```python
from build123d import *

# Parameters (mm, degrees)
F0_R     = 10.1
F1_DEPTH = 10
F2_R     = 3.75
F3_DEPTH = 10


with BuildPart() as f1:
    # F0 (on Top) → F1 (new body)
    with BuildSketch(Plane.XY):
        Circle(F0_R)
    extrude(amount=F1_DEPTH)

    # F2 (on Top) → F3 (join)
    with BuildSketch(Plane.XY):
        Circle(F2_R)
    extrude(amount=-F3_DEPTH)

    # F4 (on Front) → F5 (revolve)
    with BuildSketch(Plane.XZ):
        with BuildLine():
            Line((-3.9404258132, 0), (-10.2904258132, 0))
            Line((-10.2904258132, 0), (-10.2904258132, -9.9157679855))
            Line((-10.2904258132, -9.9157679855), (-9.0434306607, -9.9157679855))
            ThreePointArc((-9.0434306607, -9.9157679855), (-8.3038120471, -4.0254245121), (-3.9404258132, 0))
        make_face()
    revolve(axis=Axis((0, 0, -4.4246494012), (0, 0, -1)))


solid = f1.part
```
For this review, take the finished solid that the model builds, in its own axes (mm). Give positions to 0.01 mm unless a question says otherwise; leave off trailing zeros. Write each loop counter-clockwise with the first axis right and the second up, starting at its lowest first coordinate (ties: lowest second). Pieces come first, ordered by that corner, then holes.
Item 1: Wall thickness on probe 1 along Y at (x, z) = (1.5, -0.5); probe 2 along X at (y, z) = (1.25, -7.5); probe 3 along Z at (x, y) = (-8.75, -4.5): over which ranges is each line inside the solid? List them lowest first.
Item 2: The part is to be moulded in two halves that separate along X. For faces 1 (the face through (-3.746, 0.165, -4.93)), 2 (the face through (9.634, 3.034, 4.93)), 3 (the face through (0, 0, 10)), say which applies: +X half, -X half, draft (parallel to the pull), parting line (faces both ways), or undercut.
Item 3: Insertion check: P1, Ø1.5, axis at y = 8, z = -6.5, coming from the -X side; P2, Ø2, axis at y = 7, z = -5.5, coming from the -X side; P3, Ø1.5, axis at y = 1.5, z = 2.5, coming from the -X side. Each pin has a flat end and moves straight along its axis. Give the tip position at first contact, or say it passes through.
Item 4: Take a section at A-A (z = 2.25). Give the boundary of the cut face in (x, y).
Item 5: Take a section at B-B (z = -5.75). Give the number of separate pieces and of enclosed holes in the cut face, and give its area (3 significant figures).
Established:
1. probe 1: y = -10.18 to -4.72, -3.44 to 3.44, 4.72 to 10.18
1. probe 2: x = -10.21 to -9.16, -3.54 to 3.54, 9.16 to 10.21
1. probe 3: z = -9.92 to 10
2. face 1: undercut
2. face 2: parting line
2. face 3: draft
3. P1: stops at x = -7.3
3. P2: stops at x = -8.36
3. P3: stops at x = -10.07
4. outline: circle Ø20.2 at (0, 0)
5. separate pieces: 2
5. enclosed holes: 1
5. area: 124 mm2
